The model under review builds one solid part; all positions refer to its coordinate system, in mm. Round coordinates to 2 decimals unless told otherwise and drop trailing zeros. Loops run counter-clockwise (first coordinate to the right, second up) from the corner with the lowest first, then second, coordinate; pieces in that order, holes last. Notation, with made-up numbers: M -20,-31 L 33,-31 A12 cw 33,-26 Z; hole C 65.25,2 d2. An arc over 180 degrees is marked long. Answer as a JSON object with one key per item and string values. Group by question number.
Item 1: Consider section B-B (z = -106.5). Give the boundary of the cut face in (x, y).
Item 2: Consider section A-A (z = -76). Give the boundary of the cut face in (x, y).
Item 3: Insertion check: P1, Ø2, axis at y = -0.5, z = -130, coming from the +X side; P2, Ø1, axis at y = -0.5, z = -71.5, coming from the +X side; P3, Ø1, axis at x = -137, y = -1, coming from the +Z side. Each pin has a flat end and moves straight along its axis. Give the tip position at first contact, or say it passes through.
Item 4: To check wall thickness, follow line 1 (X direction, y = 1.65, z = -33.5); line 2 (X direction, y = 0.4, z = 29.5); line 3 (Z direction, x = -4.5, y = 0.5). State the ranges of each line that lie inside material, in increasing order.
```python
from build123d import *

# Parameters (mm, degrees)
F1_DEPTH = 2.38125


with BuildPart() as f1:
    # F0 (on Front) → F1 (new body, symmetric)
    with BuildSketch(Plane.XZ):
        with BuildLine():
            Line((-115.5414439804, -159.0291545598), (115.5414439804, -159.0291545598))
            Line((115.5414439804, -159.0291545598), (186.9499834696, 60.7437318397))
            add(Edge.make_bspline(
                [(-186.9499834696, 60.7437318397), (-158.5344370585, 12.5341240839), (-105.8621510044, -97.8968048071), (149.6138950392, -54.164932865), (186.9499834696, 60.7437318397)],
                knots=[0, 0, 0, 0, 0.4263853727, 1, 1, 1, 1], degree=3))
            Line((-186.9499834696, 60.7437318397), (-115.5414439804, -159.0291545598))
        make_face()
    extrude(amount=F1_DEPTH, both=True)


solid = f1.part
```
Geometry results:
{
 "1": {"outline": "M -132.61,-2.38 L 132.61,-2.38 L 132.61,2.38 L -132.61,2.38 Z"},
 "2": {"outline": "M -142.52,-2.38 L 142.52,-2.38 L 142.52,2.38 L -142.52,2.38 Z"},
 "3": {"P1": "stops at x = 125.3", "P2": "stops at x = 144.14", "P3": "stops at z = -14.24"},
 "4": {"line 1": "x = -156.33 to -116.34, 106.71 to 156.33", "line 2": "x = -176.8 to -168.68, 172.99 to 176.8", "line 3": "z = -159.03 to -62.65"}
}
